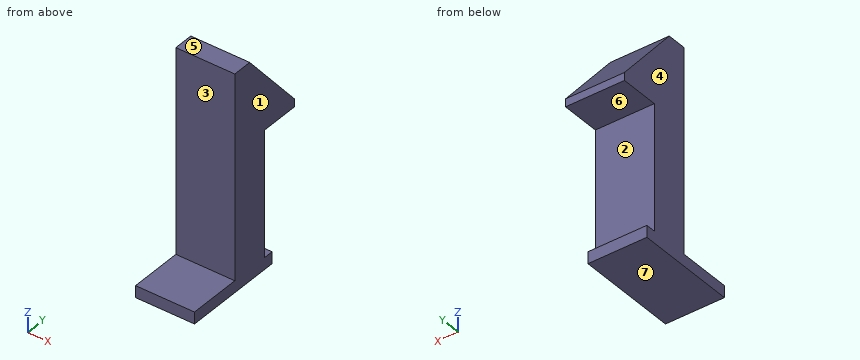
```python
from build123d import *

# Parameters (mm, degrees)
SKETCH017_W       = 3
SKETCH017_H       = 2
PAD006_DEPTH      = 4.8
PAD006_DEPTH_BACK = 1.6
PAD007_DEPTH      = 3
SKETCH020_W       = 5.2
SKETCH020_H       = 0.6
PAD008_DEPTH      = 3


with BuildPart() as part:
    # Sketch017 → Pad006 (new body, two sides)
    with BuildSketch(Plane.XY) as pad006_sk:
        Rectangle(SKETCH017_W, SKETCH017_H)
    extrude(amount=PAD006_DEPTH)
    extrude(pad006_sk.sketch, amount=-PAD006_DEPTH_BACK)

    # Sketch018 (on Face4 of Pad006) → Pad007 (join)
    with BuildSketch(Plane(origin=(-1.5, 0, 0), x_dir=(0, -1, 0), z_dir=(-1, 0, 0))):
        Polygon((1, 4.8), (-3, 4.8), (-3, 5.2), (0, 8.775261), (1, 8.775261), align=None)
    extrude(amount=-PAD007_DEPTH)

    # Sketch020 (on Face9 of Pad007) → Pad008 (join)
    with BuildSketch(Plane.YZ.offset(1.5)):
        with Locations((-1.1, -1.9)):
            Rectangle(SKETCH020_W, SKETCH020_H)
    extrude(amount=-PAD008_DEPTH)


solid = part.part
```
Part model, mm, in its own coordinate system. Face numbers are marked on the shaded views. A direction names the side the tool comes from. Coordinates: 2 decimals unless noted, no trailing zeros. Order: outer loops, then holes, each group sorted by start corner. A loop starts at its lowest first (then second) coordinate and runs counter-clockwise, first axis right, second up. Notation, with made-up numbers: (65.5, 2) -> (74.5, 2) arc R35 cw to (74.5, 40) -> close; hole circle Ø8 at (18.25, -19). An arc over 180 degrees is marked (long way). Put each result on its own line as item: value. Start each with the question number.
(1) Band-saw the part on A-A (x = -0.7). Give the cut face in (y, z).
(2) Band-saw the part on C-C (y = -2.5). Give the cut face in (x, z), then the cut area to 3 significant figures.
(3) Which spindle directions (+Z, -Z, +X, -X, +Y, -Y) get a long thin tool onto all of the face, cutting with end or side? Do the marked faces 1, 2 and 3. Say none if no direction does.
(4) Probe line 1 along Z through (x, y) = (0.95, -1.25); line 2 along Y through (x, z) = (1.25, 3); line 3 along Z through (x, y) = (0, 1.25). List the from-to ranges inside material, lowest first. Write a range as [from, to].
(5) Pin check, flat tips, straight feed: pin 1 Ø0.5 at (x, z) = (0.5, -2) entering from +Y; pin 2 Ø0.8 at (x, y) = (-0.5, -2) entering from +Z. Stop position of each tip, or through.
(6) Band-saw the part on B-B (z = 1.75). Give the cut face in (x, y).
(7) Mould opens along Z. For the marked faces 4, 5, 6 and 7 say: pulls with the +Z half, pulls with the -Z half, needs draft (parallel to the pull), parting line crosses it, or undercut.
Determined:
1. outline: (-3.7, -2.2) -> (1.5, -2.2) -> (1.5, -1.6) -> (1, -1.6) -> (1, 4.8) -> (3, 4.8) -> (3, 5.2) -> (0, 8.78) -> (-1, 8.78) -> (-1, -1.6) -> (-3.7, -1.6) -> close
2. outline: (-1.5, -2.2) -> (1.5, -2.2) -> (1.5, -1.6) -> (-1.5, -1.6) -> close
2. area: 1.80 mm²
3. face 1: +Z, -Z, +X, +Y, -Y
3. face 2: +X, -X, +Y
3. face 3: +Z, +X, -X, -Y
4. line 1: z = [-2.2, -1.6]
4. line 2: y = [-1, 1]
4. line 3: z = [-2.2, -1.6], [4.8, 7.29]
5. pin 1: stops at y = 1.5
5. pin 2: stops at z = -1.6
6. outline: (-1.5, -1) -> (1.5, -1) -> (1.5, 1) -> (-1.5, 1) -> close
7. face 4: needs draft
7. face 5: pulls with the +Z half
7. face 6: undercut
7. face 7: pulls with the -Z half
